Work out the finished part from the listing and answer in its coordinate system (mm). Face numbers are marked on the shaded views. A direction names the side the tool comes from. Give positions to 0.01 mm unless a question says otherwise; leave off trailing zeros. Order: outer loops, then holes, each group sorted by start corner. A loop starts at its lowest first (then second) coordinate and runs counter-clockwise, first axis right, second up. Notation, with made-up numbers: (-25.5, 29.25) -> (1.5, 29.25) arc R33 cw to (1.5, 58.25) -> close; hole circle Ø8 at (-31, 50.25). An arc over 180 degrees is marked (long way). Answer as CSV lines item,"result". Start each with the question number.
1. Find the intervals of material crossed by L1, parallel to X at y = -8, z = 26; L2, parallel to Y at x = 29, z = -15.5; L3, parallel to Y at x = -26, z = 21, in increasing order.
2. Flat-ended cylindrical pins translate along their axes: pin 1 (1 mm diameter, centred on x = -28.5, z = 23.5, fed in from +Y); pin 2 (3 mm diameter, centred on x = 11.5, y = -41, fed in from +Z). Find the tip coordinate at first contact, or state that the pin passes through.
3. For the marked faces 4 and 5, determine the directions among +Z, -Z, +X, -X, +Y, -Y from which every point of the face is accessible in a straight line to the end or side of a thin tool.
4. A cutting plane is placed at D-D (z = -2.5). Give the vertices of the cut face in (x, y), then the cut area to 3 significant figures.
5. A cutting plane is placed at C-C (x = -28.5). Give the vertices of the cut face in (y, z), then the cut area to 3 significant figures.
6. A cutting plane is placed at A-A (z = 21). Give the vertices of the cut face in (x, y).
7. For a pull along X with two mould halves and no side action, classify the marked faces 1, 2 and 3 as released by +X, released by -X, zero draft, split by the parting line, or undercut.
8. A cutting plane is placed at B-B (y = 6.5). Give the vertices of the cut face in (x, z), then the cut area to 3 significant figures.
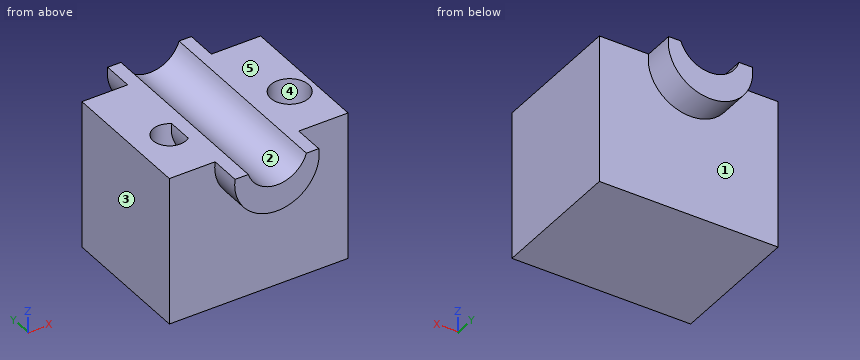
from build123d import *

# Parameters (mm, degrees)
F1_DEPTH = 42.418
F2_DEPTH = 25.4
F3_R     = 8.2419293277
F3_R_2   = 9.4983562565
F4_DEPTH = 25.4
F6_DEPTH = 15.494
F7_DEPTH = 98.806


with BuildPart() as f1:
    # F0 (on Front) → F1 (new body)
    with BuildSketch(Plane.XZ):
        with BuildLine():
            Line((-44.7798408568, -37.1997542679), (44.7798408568, -37.1997542679))
            Line((44.7798408568, -37.1997542679), (44.7798408568, 37.1997542679))
            Line((44.7798408568, 37.1997542679), (13.8912415132, 37.1997542679))
            ThreePointArc((13.8912415132, 37.1997542679), (-0.6620394997, 26.4881938236), (-15.2153205127, 37.1997542679))
            Line((-15.2153205127, 37.1997542679), (-44.7798408568, 37.1997542679))
            Line((-44.7798408568, 37.1997542679), (-44.7798408568, -37.1997542679))
        make_face()
    extrude(amount=F1_DEPTH)

    # F2 (add): a face of the model
    f2_faces = [f1.faces().sort_by_distance(p)[0] for p in [
        (0.023550187, 0, -1.1650746178),
    ]]
    extrude(f2_faces, amount=F2_DEPTH)

    # F3 (on face) → F4 (cut)
    with BuildSketch(Plane.XY.offset(37.1997542679)):
        with Locations((-27.1278675646, -15.2127910405)):
            Circle(F3_R)
        with Locations((32.7657014132, -15.7461762428)):
            Circle(F3_R_2)
    extrude(amount=-F4_DEPTH, mode=Mode.SUBTRACT)

    # F5 (on face) → F6 (join)
    with BuildSketch(Plane(origin=(0, 25.4, 0), x_dir=(-1, 0, 0), z_dir=(0, 1, 0))):
        with BuildLine():
            Line((-13.8912415132, 37.1997542679), (-20.0768597424, 37.1997542679))
            ThreePointArc((-20.0768597424, 37.1997542679), (0.892303884, 13.1906008043), (21.8614675105, 37.1997542679))
            Line((21.8614675105, 37.1997542679), (15.2153205127, 37.1997542679))
            ThreePointArc((15.2153205127, 37.1997542679), (0.6620394997, 26.4881938236), (-13.8912415132, 37.1997542679))
        make_face()
    extrude(amount=F6_DEPTH)

    # F7 (add): a face of the model
    f7_faces = [f1.faces().sort_by_distance(p)[0] for p in [
        (-0.9809266979, 40.894, 24.6318150019),
    ]]
    extrude(f7_faces, amount=-F7_DEPTH)


solid = f1.part
Answer sheet:
1,L1,"x = -44.78 to -31.12, -23.14 to 27.27, 38.26 to 44.78"
1,L2,"y = -42.42 to 25.4"
1,L3,"y = -42.42 to -23.38, -7.05 to 25.4"
2,pin 1,"stops at y = 25.4"
2,pin 2,"stops at z = 34.97"
3,face 4,"+Z"
3,face 5,"+Z, +X, -X, +Y, -Y"
4,outline,"(-44.78, -42.42) -> (44.78, -42.42) -> (44.78, 25.4) -> (-44.78, 25.4) -> close"
4,area,"6,070 mm^2"
5,outline,"(-42.42, -37.2) -> (25.4, -37.2) -> (25.4, 37.2) -> (-7.09, 37.2) -> (-7.09, 11.8) -> (-23.34, 11.8) -> (-23.34, 37.2) -> (-42.42, 37.2) -> close"
5,area,"4,630 mm^2"
6,outline,"(-44.78, -42.42) -> (-17.31, -42.42) -> (-17.31, -57.91) -> (15.53, -57.91) -> (15.53, -42.42) -> (44.78, -42.42) -> (44.78, 25.4) -> (15.53, 25.4) -> (15.53, 40.89) -> (-17.31, 40.89) -> (-17.31, 25.4) -> (-44.78, 25.4) -> close; hole circle Ø16.48 at (-27.13, -15.21); hole circle Ø19 at (32.77, -15.75)"
7,face 1,"zero draft"
7,face 2,"undercut"
7,face 3,"released by -X"
8,outline,"(-44.78, -37.2) -> (44.78, -37.2) -> (44.78, 37.2) -> (13.89, 37.2) arc R15.24 cw to (-15.22, 37.2) -> (-44.78, 37.2) -> close"
8,area,"6,430 mm^2"
